The listing builds one solid part. Answer for the finished solid, in the listing's coordinates (mm). A direction names the side the tool comes from. Coordinates: 2 decimals unless noted, no trailing zeros. Loops run counter-clockwise (first coordinate to the right, second up) from the corner with the lowest first, then second, coordinate; pieces in that order, holes last. Notation, with made-up numbers: (-36.5, 65) - (1.5, 65) arc R28 cw to (1.5, 91) - close; hole circle Ø10 at (18.25, -3.75). An arc over 180 degrees is marked (long way). Return JSON: item names as keys, results as strings. Group by question number.
1. The mould has two halves that part along X. Classify faces 4 (the face through (13.112, 2.24, 29.237)), 5 (the face through (21.763, 2.24, 11.337)), 6 (the face through (0, 3, 17)): pulls with the +X half, pulls with the -X half, needs draft (parallel to the pull), parting line crosses it, or undercut.
2. Find the intervals of material crossed by line 1 along Z through (x, y) = (9.5, 2); line 2 along X through (y, z) = (2, 1.65); line 3 along Y through (x, z) = (1.9, 5), in increasing order.
3. Section B-B (y = 2) is taken. State how many separate pieces and enclosed holes the cut face has, and give its area (3 significant figures).
4. Each of these flat-tipped pins is pushed along its axis until it touches: P1, Ø0.9, axis at x = 25, z = 19, coming from the +Y side; P2, Ø1.4, axis at x = 5, y = 2, coming from the -Z side. Where does it stop, or does it pass through?
5. Section C-C (x = 22.5) is taken. Write down the section's boundary in (y, z), and give its area (3 significant figures).
6. Section D-D (z = 20) is taken. Write down the section's boundary in (x, y) (3 decimals).
7. Section A-A (x = 2) is taken. Write down the section's boundary in (y, z).
8. Which of the six approach directions +Z, -Z, +X, -X, +Y, -Y give full straight-line access (tool end or side, diameter ignored) to faces 1 (the face through (25, 4, 17)), 2 (the face through (19.85, 3.81, 17.74)), 3 (the face through (2.535, 1.694, 16.761))?
Autodesk Inventor part; units mm, degrees
ref_plane "YZ Plane" through (0, 0, 0) normal (1, 0, 0) x (0, 1, 0)
ref_plane "XZ Plane" through (0, 0, 0) normal (0, 1, 0) x (-1, 0, 0)
ref_plane "XY Plane" through (0, 0, 0) normal (0, 0, 1) x (1, 0, 0)
sketch "スケッチ1" plane through (0, 0, 0) normal (0, 0, 1) x (1, 0, 0)
  line L0 (0, 16.5) -> (26, 16.5)
  line L1 (26, 16.5) -> (26, 0)
  line L2 (26, 0) -> (0, 0)
  line L3 (0, 0) -> (0, 16.5)
  circle A0 centre (13, 16.5) radius 12.5
  line L4 (13, 4) -> (26, 4)
  arc A1 (0, 10.25) -> (13, 4) centre (13, 20.645) ccw
  line L5 (13, 4) -> (0, 4)
  point P0 (25.5, 16.5)
  point P1 (0.5, 16.5)
  dimension "d0" = 25
  dimension "d1" = 26
  dimension "d2" = 16.5
  dimension "d8" = 6.25
  dimension "d9" = 6.25
extrude "押し出し1" add sketch "スケッチ1" along normal blind 35 contours L5 L3 A1 | L4 L1 L2 L3 L5
fillet "フィレット4" radius 2 1 edges at (0, 10.25, 17.5)
sketch "スケッチ2" plane through (26, 0, 0) normal (1, 0, 0) x (0, 0, -1)
  circle A0 centre (-30, 2) radius 0.8
  circle A1 centre (-5, 2) radius 0.8
  line L0 (0, 0) -> (-35, 0)
  line L1 (-35, 0) -> (-35, 4)
  line L2 (0, 0) -> (0, 4)
  circle A2 centre (-17.5, 2) radius 0.8
  dimension "d11" = 1.6
  dimension "d12" = 1.6
  dimension "d13" = 2
  dimension "d14" = 5
  dimension "d15" = 5
  dimension "d26" = 12.5
  dimension "d27" = 12.5
extrude "押し出し2" cut sketch "スケッチ2" against normal through all
sketch "スケッチ3" plane through (0, 0, 35) normal (0, 0, 1) x (1, 0, 0)
  circle A0 centre (2, 5.5906) radius 0.8
  circle A1 centre (5, 2) radius 0.8
  circle A2 centre (21, 2) radius 0.8
  line L0 (0, 0) -> (26, 0)
  line L1 (26, 0) -> (26, 4)
  line L2 (0, 5.5906) -> (0, 0)
  arc A3 (3.1799, 7.2054) -> (0, 5.5906) centre (2, 5.5906) ccw
  dimension "d18" = 1.6
  dimension "d19" = 1.6
  dimension "d20" = 1.6
  dimension "d21" = 2
  dimension "d22" = 5
  dimension "d23" = 5
extrude "押し出し3" cut sketch "スケッチ3" against normal through all
sketch "スケッチ4" plane through (0, 0, 35) normal (0, 0, 1) x (1, 0, 0)
  arc A0 (3.1799, 7.2054) -> (13, 4) centre (13, 20.645) ccw
  circle A1 centre (13, 16.5) radius 12.5 construction
  line L0 (13, 16.5) -> (13, 4) construction
  circle A2 centre (13, 16.5) radius 13.5
  point P0 (0, 0)
  dimension "d30" = 25
  dimension "d31" = 27
extrude "押し出し4" cut sketch "スケッチ4" against normal through all
fillet "フィレット5" radius 50 1 edges at (18.099, 4, 17.5)
equation "\"d8\" = d9"
equation "\"d26\" = d27"
properties part number "hipjoint_toleg_middle"
The answers:
{
 "1": {"face 4": "needs draft", "face 5": "undercut", "face 6": "pulls with the -X half"},
 "2": {"line 1": "z = 0 to 4.2, 5.8 to 16.7, 18.3 to 29.2, 30.8 to 35", "line 2": "x = 0 to 4.2, 5.8 to 20.2, 21.8 to 26", "line 3": "y = 0 to 1.2, 2.8 to 4.8, 6.38 to 7.59"},
 "3": {"separate pieces": "12", "enclosed holes": "0", "area": "689 mm2"},
 "4": {"P1": "stops at y = 4", "P2": "passes through"},
 "5": {"outline": "(0, 0) - (3.97, 0) - (3.97, 35) - (0, 35) - close; hole circle Ø1.6 at (2, 5); hole circle Ø1.6 at (2, 17.5); hole circle Ø1.6 at (2, 30)", "area": "133 mm2"},
 "6": {"outline": "(0, 0) - (26, 0) - (26, 4) - (24.225, 4) arc R50 ccw to (15.386, 3.213) arc R13.5 cw to (3.275, 7.136) arc R16.645 cw to (3.18, 7.205) arc R2 ccw to (0, 5.591) - close; hole circle Ø1.6 at (2, 5.591); hole circle Ø1.6 at (5, 2); hole circle Ø1.6 at (21, 2)"},
 "7": {"outline": "(0, 0) - (4.79, 0) - (4.79, 35) - (0, 35) - close; (6.39, 0) - (7.59, 0) - (7.59, 35) - (6.39, 35) - close; hole circle Ø1.6 at (2, 5); hole circle Ø1.6 at (2, 17.5); hole circle Ø1.6 at (2, 30)"},
 "8": {"face 1": "+Z, -Z, +X, +Y", "face 2": "+Z, -Z, +Y", "face 3": "+X, -X"}
}
